For this review, take the finished solid that the model builds, in its own axes (mm). A direction names the side the tool comes from. Coordinates: 2 decimals unless noted, no trailing zeros. Loops run counter-clockwise (first coordinate to the right, second up) from the corner with the lowest first, then second, coordinate; pieces in that order, holes last. Notation, with made-up numbers: M 84,-34.5 L 139,-34.5 A27 ccw 139,-11.5 Z; hole C 82.5,53 d1. An arc over 180 degrees is marked long. Write item = value, one per line.
from build123d import *

# Parameters (mm, degrees)
F0_R     = 2.5
F1_DEPTH = 3


with BuildPart() as f1:
    # F0 (on Top) → F1 (new body)
    with BuildSketch(Plane.XY):
        with BuildLine():
            ThreePointArc((-7.5958592746, 30.447376996), (-7.2954421995, 29.7607968689), (-7.6664191036, 29.1096295889))
            add(Edge.make_bspline(
                [(-7.6664191036, 29.1096295889), (-55.464118768, -2.7410070687), (-6.5156015718, -29.8104974613)],
                knots=[0.3967115562, 0.3967115562, 0.3967115562, 2.8069981351, 2.8069981351, 2.8069981351], degree=2, weights=[1, 0.357559236, 1]))
            ThreePointArc((-6.5156015718, -29.8104974613), (31.5120821846, -17.9102618156), (17.8725918917, 19.5288172976))
            ThreePointArc((17.8725918917, 19.5288172976), (17.2999162533, 19.3489700798), (17.4003215692, 18.7571751989))
            ThreePointArc((17.4003215692, 18.7571751989), (26.4978981224, -1.3229207129), (16.0357766574, -20.7270482486))
            ThreePointArc((16.0357766574, -20.7270482486), (15.418361067, -20.6961037556), (15.3029208356, -20.0887874247))
            add(Edge.make_bspline(
                [(15.3029208356, -20.0887874247), (32.3088785024, 12.6887970766), (7.6664191036, 29.1096295889)],
                knots=[4.022421846, 4.022421846, 4.022421846, 5.886473751, 5.886473751, 5.886473751], degree=2, weights=[1, 0.5962087126, 1]))
            ThreePointArc((7.6664191036, 29.1096295889), (7.2954421995, 29.7607968689), (7.5958592746, 30.447376996))
            ThreePointArc((7.5958592746, 30.447376996), (11.762218697, 37.8714882822), (9.8957824129, 46.1776543547))
            Line((9.8957824129, 46.1776543547), (10.4372317457, 54.1401412002))
            ThreePointArc((10.4372317457, 54.1401412002), (10.142102083, 54.646218012), (9.5627349759, 54.5593329591))
            Line((9.5627349759, 54.5593329591), (5.0160304443, 50.3683832584))
            ThreePointArc((5.0160304443, 50.3683832584), (0, 51.478518162), (-5.0160304443, 50.3683832584))
            Line((-5.0160304443, 50.3683832584), (-9.5627349759, 54.5593329591))
            ThreePointArc((-9.5627349759, 54.5593329591), (-10.142102083, 54.646218012), (-10.4372317457, 54.1401412002))
            Line((-10.4372317457, 54.1401412002), (-9.8957824129, 46.1776543547))
            ThreePointArc((-9.8957824129, 46.1776543547), (-11.762218697, 37.8714882822), (-7.5958592746, 30.447376996))
        make_face()
        with Locations((0, -25.7397647947)):
            Circle(F0_R, mode=Mode.SUBTRACT)
    extrude(amount=F1_DEPTH)


solid = f1.part
Q1. For pin 1 Ø1 at (x, z) = (18.5, 2) entering from +Y, flat-tipped, find the tip position at first contact; note if it passes through.
Solved:
pin_1 = 19.47
Q2. Add section C-C (x = 28). Write out the cut boundary in (y, z), and give its area (3 significant figures).
Solved:
outline = M -23.31,0 L 11.91,0 L 11.91,3 L -23.31,3 Z
area = 106 mm²
Q3. Machinability: for faces 1 (the face through (-10.17, 50.21, 1.48)), 2 (the face through (26.507, -1.003, 1.479)), 3 (the face through (11.744, 37.751, 1.479)), 4 (the face through (-7.258, 52.435, 1.479)), 5 (the face through (6, 4, 0)), which of the approach directions +Z, -Z, +X, -X, +Y, -Y give a long, thin tool a straight path to every point of the face, cutting with its end or side? Answer none if there is none.
Solved:
face_1 = +Z, -Z, -X
face_2 = +Z, -Z
face_3 = +Z, -Z, +X
face_4 = +Z, -Z, +Y
face_5 = -Z, +X, -X, +Y, -Y
Q4. Add section A-A (x = 1.5). Write out the cut boundary in (y, z), and give its area (3 significant figures).
Solved:
outline = M -32.73,0 L -27.74,0 L -27.74,3 L -32.73,3 Z; M -23.74,0 L 51.38,0 L 51.38,3 L -23.74,3 Z
area = 240 mm²
Q5. Draft analysis for pull direction X (two halves, no side actions). For faces 6 (the face through (0.07, 51.48, 1.48)), 7 (the face through (7.32, 52.49, 1.48)), 8 (the face through (-11.78, 37.99, 1.48)), 9 (the face through (10.163, 50.103, 1.479)), state which applies: +X half, -X half, draft (parallel to the pull), parting line (faces both ways), or undercut.
Solved:
face_6 = undercut
face_7 = undercut
face_8 = -X half
face_9 = +X half
Q6. Add section B-B (y = 44). Write out the cut boundary in (x, z), and give its area (3 significant figures).
Solved:
outline = M -11.04,0 L 11.04,0 L 11.04,3 L -11.04,3 Z
area = 66.2 mm²
Q7. For line 1 along X through (y, z) = (17, 0.75); line 2 along X through (y, z) = (-9, 2.6); line 3 along Y through (x, z) = (22.5, 0.75), list the stretches that pass through material, from the lowest coordinate up.
Solved:
line_1 = -16.72 to 16.72, 19.33 to 22.42
line_2 = -19.02 to 19.02, 25 to 34.17
line_3 = -28.35 to -14, 13.07 to 16.94
